Here's how the part is built. I have some questions about the finished solid (model axes, mm). A direction names the side the tool comes from. Coordinates: 2 decimals unless noted, no trailing zeros. Loops run counter-clockwise (first coordinate to the right, second up) from the corner with the lowest first, then second, coordinate; pieces in that order, holes last. Notation, with made-up numbers: (-35, 37) -> (-13, 37) arc R18 ccw to (-13, 50) -> close; hole circle Ø6 at (75, 13.25). An arc over 180 degrees is marked (long way). Answer as a JSON object with one key per item and string values. Group by question number.
Q1. I'm going to push flat-ended pins straight in: pin 1 (3 mm diameter, centred on x = -10, z = 122.5, fed in from +Y); pin 2 (2.5 mm diameter, centred on x = -0.85, z = 194.9, fed in from +Y). Where does each tip first touch, or does it pass through?
Q2. Thinking about a two-plate mould opening in Y: for faces 1 (the cylindrical face through (-4.729, 22.966, 112.99)), 2 (the cylindrical face through (-9.91, 26.028, 120.916)), 3 (the flat face through (-5, 19, 119.399)), 4 (the flat face through (-1, 24, 195)), which applies, released by +Y, released by -Y, zero draft, split by the parting line, or undercut?
Q3. I want a section at B-B on x = 3.5. Write out the boundary of the cut face in (y, z), then the cut area to 3 significant figures.
Q4. I want a section at A-A on y = 19. Write out the boundary of the cut face in (x, z).
Q5. I need wall thicknesses on line 1 (Z direction, x = -9.65, y = 25.5); line 2 (Y direction, x = -5.25, z = 109); line 3 (Z direction, x = -3.5, y = 13.5). Which ranges of each line are inside material? Lowest first, please.
Q6. On a 3-axis mill with a long thin cutter (end or side, diameter ignored), from which of +Z, -Z, +X, -X, +Y, -Y can I reach the whole of each face in a straight line? I mean faces 5 (the flat face through (5.5, 19, 160)), 6 (the flat face through (-1, 24, 123)), 7 (the flat face through (-5, 25, 119.399)). Say none if no direction works.
```python
from build123d import *

# Parameters (mm, degrees)
BOSS_EXTRUDE6_START = 10
SKETCH22_W          = 21.5
SKETCH22_H          = 80
BOSS_EXTRUDE6_DEPTH = 18
SKETCH23_R          = 2
CUT_EXTRUDE9_DEPTH  = 4
SKETCH24_R          = 5.5
SKETCH24_R_2        = 4
BOSS_EXTRUDE7_DEPTH = 13


with BuildPart() as part:
    # Sketch22 → Boss-Extrude6 (new body)
    with BuildSketch(Plane(origin=(0, 0, 0), x_dir=(1, 0, 0), z_dir=(0, 1, 0)).offset(BOSS_EXTRUDE6_START)):
        with Locations((-5.25, -159.399454256)):
            Rectangle(SKETCH22_W, SKETCH22_H)
    extrude(amount=BOSS_EXTRUDE6_DEPTH)

    # Sketch23 → Cut-Extrude9 (cut)
    with BuildSketch(Plane(origin=(0, 28, 0), x_dir=(1, 0, 0), z_dir=(0, 1, 0))):
        with Locations((-9.65, -122.899454256)):
            Circle(SKETCH23_R)
        with Locations((-0.85, -122.899454256)):
            Circle(SKETCH23_R)
        with Locations((-0.85, -194.899454256)):
            Circle(SKETCH23_R)
        with Locations((-9.65, -194.899454256)):
            Circle(SKETCH23_R)
    extrude(amount=-CUT_EXTRUDE9_DEPTH, mode=Mode.SUBTRACT)

    # Sketch24 → Boss-Extrude7 (add)
    with BuildSketch(Plane(origin=(0, 0, 119.399454256), x_dir=(-1, 0, 0), z_dir=(0, 0, -1))):
        with Locations((5.25, 19)):
            Circle(SKETCH24_R)
        with Locations((5.25, 19)):
            Circle(SKETCH24_R_2, mode=Mode.SUBTRACT)
    extrude(amount=BOSS_EXTRUDE7_DEPTH)


solid = part.part
```
Result set:
{
 "1": {"pin 1": "stops at y = 28", "pin 2": "stops at y = 24"},
 "2": {"face 1": "undercut", "face 2": "zero draft", "face 3": "undercut", "face 4": "released by +Y"},
 "3": {"outline": "(10, 119.4) -> (28, 119.4) -> (28, 199.4) -> (10, 199.4) -> close", "area": "1,440 mm²"},
 "4": {"outline": "(-16, 119.4) -> (-10.75, 119.4) -> (-10.75, 106.4) -> (-9.25, 106.4) -> (-9.25, 119.4) -> (-1.25, 119.4) -> (-1.25, 106.4) -> (0.25, 106.4) -> (0.25, 119.4) -> (5.5, 119.4) -> (5.5, 199.4) -> (-16, 199.4) -> close"},
 "5": {"line 1": "z = 119.4 to 120.9, 124.9 to 192.9, 196.9 to 199.4", "line 2": "y = 13.5 to 15, 23 to 24.5", "line 3": "z = 119.4 to 199.4"},
 "6": {"face 5": "+Z, -Z, +X, +Y, -Y", "face 6": "+Y", "face 7": "-Z"}
}
